The listing builds one solid part. Answer for the finished solid, in the listing's coordinates (mm). Give positions to 0.01 mm unless a question says otherwise; leave off trailing zeros. Write each loop counter-clockwise with the first axis right and the second up, starting at its lowest first coordinate (ties: lowest second). Pieces come first, ordered by that corner, then holes.
```python
from build123d import *

# Parameters (mm, degrees)
SKETCH1_W               = 17.5
SKETCH1_H               = 25
SKETCH1_W_2             = 25
SKETCH1_H_2             = 230
SKETCH1_H_3             = 20
BOSS_EXTRUDE1_DEPTH     = 3
CUT_EXTRUDE1_DEPTH      = 121.996900787
CUT_EXTRUDE1_DEPTH_BACK = 121.996900787
SKETCH2_R               = 1.5
CUT_EXTRUDE2_DEPTH      = 121.996900787
CUT_EXTRUDE2_DEPTH_BACK = 121.996900787
SKETCH3_R               = 4
SKETCH3_W               = 15
SKETCH3_H               = 10


with BuildPart() as part:
    # Sketch1 → Boss-Extrude1 (new body)
    with BuildSketch(Plane(origin=(0, 0, 0), x_dir=(1, 0, 0), z_dir=(0, 1, 0))):
        with Locations((21.25, 53.5)):
            Rectangle(SKETCH1_W, SKETCH1_H)
        Rectangle(SKETCH1_W_2, SKETCH1_H_2)
        with Locations((-21.25, 53.5)):
            Rectangle(SKETCH1_W, SKETCH1_H)
        with Locations((21.25, 102.5)):
            Rectangle(SKETCH1_W, SKETCH1_H)
        with Locations((-21.25, 102.5)):
            Rectangle(SKETCH1_W, SKETCH1_H)
        with Locations((-25, -105)):
            Rectangle(SKETCH1_W_2, SKETCH1_H_3)
        with Locations((25, -105)):
            Rectangle(SKETCH1_W_2, SKETCH1_H_3)
    extrude(amount=BOSS_EXTRUDE1_DEPTH)

    # Sketch2 → Cut-Extrude1 (cut, two sides: drawn at the far end of the back side and taken through both)
    with BuildSketch(Plane(origin=(0, 3, 0), x_dir=(1, 0, 0), z_dir=(0, 1, 0)).offset(-CUT_EXTRUDE1_DEPTH_BACK)):
        with Locations(Location((-21.25, 102.5, 0), (0, 0, 270))):
            Circle(SKETCH2_R)
        with Locations(Location((21.25, 102.5, 0), (0, 0, 270))):
            Circle(SKETCH2_R)
        with Locations(Location((-21.25, 53.5, 0), (0, 0, 270))):
            Circle(SKETCH2_R)
        with Locations(Location((21.25, 53.5, 0), (0, 0, 270))):
            Circle(SKETCH2_R)
    extrude(amount=CUT_EXTRUDE1_DEPTH + CUT_EXTRUDE1_DEPTH_BACK, mode=Mode.SUBTRACT)

    # Sketch3 → Cut-Extrude2 (cut, two sides: drawn at the far end of the back side and taken through both)
    with BuildSketch(Plane(origin=(0, 3, 0), x_dir=(1, 0, 0), z_dir=(0, 1, 0)).offset(-CUT_EXTRUDE2_DEPTH_BACK)):
        with Locations(Location((-25, -105, 0), (0, 0, 270))):
            Circle(SKETCH3_R)
        with Locations(Location((25, -105, 0), (0, 0, 270))):
            Circle(SKETCH3_R)
        with Locations((0, -105)):
            Rectangle(SKETCH3_W, SKETCH3_H)
    extrude(amount=CUT_EXTRUDE2_DEPTH + CUT_EXTRUDE2_DEPTH_BACK, mode=Mode.SUBTRACT)


solid = part.part
```
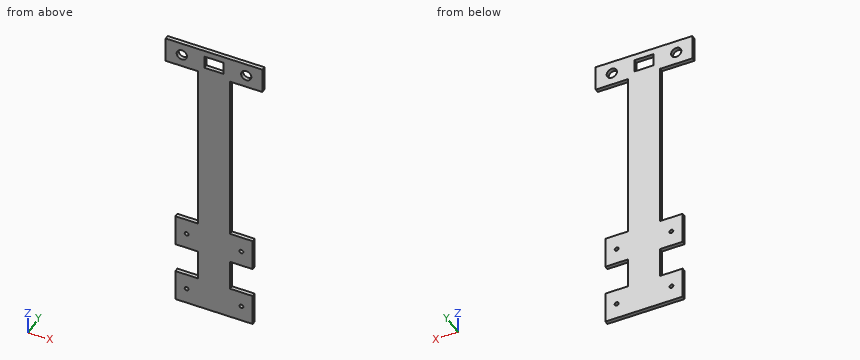
Item 1: A cutting plane is placed at A-A, the plane y = 2.15. Count the separate pieces of the cut face and the enclosed holes in it, plus the area to 3 significant figures.
Conclusion:
separate pieces: 1
enclosed holes: 7
area: 8,220 mm2
Item 2: A cutting plane is placed at B-B, the plane x = -25. Give the vertices of the cut face in (y, z), plus the area to 3 significant figures.
Conclusion:
outline: (0, -115) - (3, -115) - (3, -90) - (0, -90) - close; (0, -66) - (3, -66) - (3, -41) - (0, -41) - close; (0, 95) - (3, 95) - (3, 101) - (0, 101) - close; (0, 109) - (3, 109) - (3, 115) - (0, 115) - close
area: 186 mm2
Item 3: Each of these flat-tipped pins is pushed along its axis until it touches: P1, Ø1.5, axis at y = 1.5, z = 33, coming from the -X side; P2, Ø1, axis at y = 0.5, z = 59.5, coming from the +X side; P3, Ø1.5, axis at x = 31, y = 1, coming from the -Z side. Where does it stop, or does it pass through?
Conclusion:
P1: stops at x = -12.5
P2: stops at x = 12.5
P3: stops at z = 95
Item 4: Consider probe 1 along Z at (x, y) = (29.5, 1.95); probe 2 along X at (y, z) = (1.15, -102.5); probe 3 along Z at (x, y) = (-25, 1.85). Determine where each line is inside the solid, lowest interval first.
Conclusion:
probe 1: z = -115 to -90, -66 to -41, 95 to 115
probe 2: x = -30 to -22.75, -19.75 to 19.75, 22.75 to 30
probe 3: z = -115 to -90, -66 to -41, 95 to 101, 109 to 115
Item 5: A cutting plane is placed at D-D, the plane z = 19.5. Give the vertices of the cut face in (x, y).
Conclusion:
outline: (-12.5, 0) - (12.5, 0) - (12.5, 3) - (-12.5, 3) - close
Item 6: A cutting plane is placed at C-C, the plane z = 105. Give the vertices of the cut face in (x, y).
Conclusion:
outline: (-37.5, 0) - (-29, 0) - (-29, 3) - (-37.5, 3) - close; (-21, 0) - (-7.5, 0) - (-7.5, 3) - (-21, 3) - close; (7.5, 0) - (21, 0) - (21, 3) - (7.5, 3) - close; (29, 0) - (37.5, 0) - (37.5, 3) - (29, 3) - close
